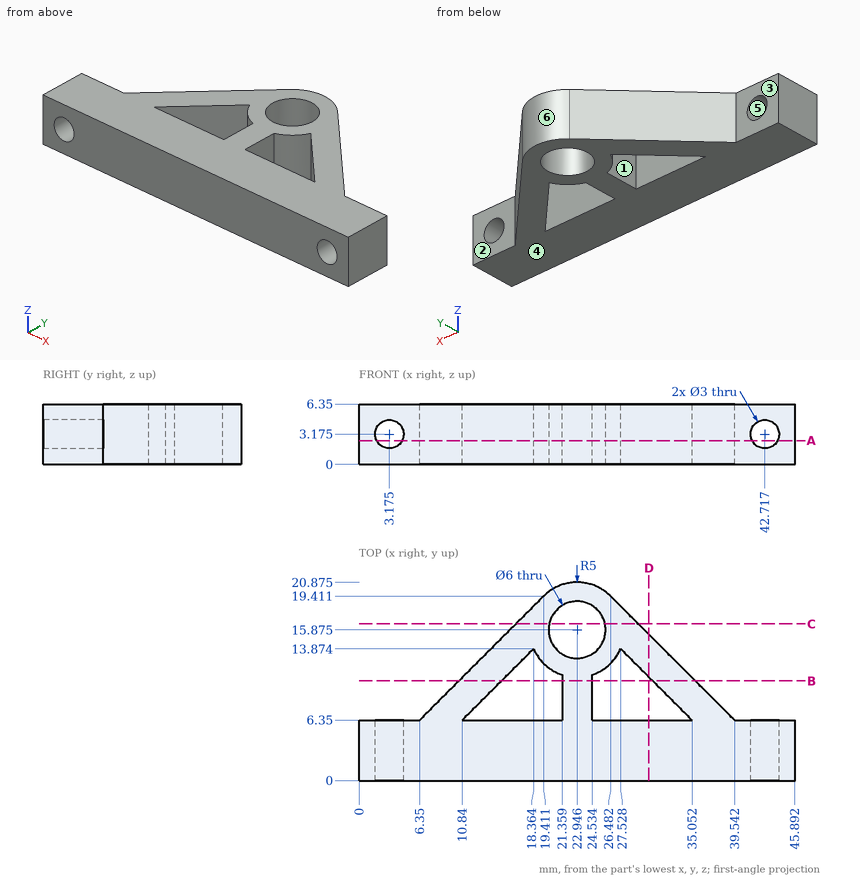
Geometry check sheet. Reference: drawing and pictorial views, mm from the part's lowest x, y, z. A direction names the side the tool comes from. Round coordinates to 2 decimals unless told otherwise and drop trailing zeros. Order: outer loops, then holes, each group sorted by start corner. A loop starts at its lowest first (then second) coordinate and runs counter-clockwise, first axis right, second up. Notation, with made-up numbers: (-37, 31) -> (19, 31) arc R34 cw to (19, 70) -> close; hole circle Ø6 at (83, -11.5). An arc over 180 degrees is marked (long way). One line per item, written item: value. Start each with the question number.
Q1. Set-up check for the marked faces 1, 2 and 3: record each of +Z, -Z, +X, -X, +Y, -Y from which the full face is reachable in a straight line by a thin tool's end or side.
Q2. Cross-section at A-A (z = 2.5). Give the number of separate pieces and of enclosed holes in the cut face, and give its area (3 significant figures).
Q3. Cross-section at D-D (x = 30.5). Record the boundary of the cut face in (y, z).
Q4. Cross-section at B-B (y = 10.5). Record the boundary of the cut face in (x, z).
Q5. Thickness scan on line 1 (X direction, y = 2, z = 3.25) (1 decimal); line 2 (X direction, y = 6, z = 2.5) (1 decimal); line 3 (X direction, y = 17.5, z = 4.25) (1 decimal). Record the ranges inside material, lowest first.
Q6. Mould release check, pull along Z, two halves, no side actions. Record for the marked faces 4, 5 and 6: pulls with the +Z half, pulls with the -Z half, needs draft (parallel to the pull), parting line crosses it, or undercut.
Q7. Cross-section at C-C (y = 16.5). Record the boundary of the cut face in (x, z), and give its area (3 significant figures).
Q8. Gauge pin test, flat ends, axial feed: pin 1 Ø3 at (x, z) = (17.5, 4) entering from +Y; pin 2 Ø1.4 at (y, z) = (10, 2) entering from +X; pin 3 Ø1.4 at (y, z) = (9, 1.5) entering from -X; pin 4 Ø5 at (x, y) = (22.95, 15.88) entering from +Z. Record the tip position at first contact, or that the pin passes through.
Completed:
1. face 1: +Z, -Z
1. face 2: +Z, -Z, +X, +Y
1. face 3: +Z, -Z, -X, +Y
2. separate pieces: 3
2. enclosed holes: 3
2. area: 408 mm²
3. outline: (0, 0) -> (6.35, 0) -> (6.35, 6.35) -> (0, 6.35) -> close; (10.9, 0) -> (15.39, 0) -> (15.39, 6.35) -> (10.9, 6.35) -> close
4. outline: (10.5, 0) -> (14.99, 0) -> (14.99, 6.35) -> (10.5, 6.35) -> close; (21.36, 0) -> (24.53, 0) -> (24.53, 6.35) -> (21.36, 6.35) -> close; (30.9, 0) -> (35.39, 0) -> (35.39, 6.35) -> (30.9, 6.35) -> close
5. line 1: x = 0 to 1.7, 4.7 to 41.2, 44.2 to 45.9
5. line 2: x = 0 to 1.8, 4.5 to 41.4, 44.1 to 45.9
5. line 3: x = 17.5 to 20.4, 25.5 to 28.4
6. face 4: pulls with the -Z half
6. face 5: undercut
6. face 6: needs draft
7. outline: (16.5, 0) -> (20.01, 0) -> (20.01, 6.35) -> (16.5, 6.35) -> close; (25.88, 0) -> (29.39, 0) -> (29.39, 6.35) -> (25.88, 6.35) -> close
7. area: 44.6 mm²
8. pin 1: stops at y = 19
8. pin 2: stops at x = 36.59
8. pin 3: stops at x = 8.3
8. pin 4: passes through
